```python
from build123d import *

# Parameters (mm, degrees)
CUT_EXTRUDE_2_DEPTH      = 0.5
PATTERN_CIRCULAR_1_COUNT = 2
PATTERN_CIRCULAR_1_ANGLE = 90
CUT_EXTRUDE_3_REACH      = 23.556
CUT_EXTRUDE_3_END_RADIUS = 6.5
SKETCH_4_R               = 0.85


with BuildPart() as part:
    # 草图1 → 旋转1 (revolve)
    with BuildSketch(Plane.XY, mode=Mode.PRIVATE) as revolve_1_sk:
        with BuildLine():
            Line((0, 0), (0, 2))
            Line((0, 2), (-20, 2))
            Line((-20, 2), (-20, 4))
            Line((-20, 4), (-21.524428901, 4))
            ThreePointArc((-21.524428901, 4), (-21.705500393, 3.956669476), (-21.847342271, 3.836065574))
            ThreePointArc((-21.847342271, 3.836065574), (-22.778904626, 2.017706029), (-23.1, 0))
            Line((-23.1, 0), (0, 0))
        make_face()
    revolve(revolve_1_sk.sketch.rotate(Axis((0, 0, 0), (-1, 0, 0)), 90), axis=Axis((0, 0, 0), (-1, 0, 0)))

    # 草图3 → 切除-拉伸2 (cut, symmetric)
    with BuildSketch(Plane.XY):
        Polygon((-20.8, -1), (-23.8, -2.495744824), (-23.8, 2.495744824), (-20.8, 1), align=None)
    cut_extrude_2 = extrude(amount=CUT_EXTRUDE_2_DEPTH, both=True, mode=Mode.SUBTRACT)

    # 阵列(圆周)1: 切除-拉伸2 ×2 about axis
    pattern_circular_1_axis = Axis((0, 0, 0), (1, 0, 0))
    for i in range(1, PATTERN_CIRCULAR_1_COUNT):
        add(cut_extrude_2.rotate(pattern_circular_1_axis, i * PATTERN_CIRCULAR_1_ANGLE / (PATTERN_CIRCULAR_1_COUNT - 1)), mode=Mode.SUBTRACT)

    # 切除-拉伸3: up to this sphere (the profile starts inside it)
    cut_extrude_3_end = Location((-16.6, 0, 0)) * Sphere(CUT_EXTRUDE_3_END_RADIUS, mode=Mode.PRIVATE)
    # 草图4 → 切除-拉伸3 (cut, up to the surface)
    with BuildSketch(Plane.ZY.offset(20.8), mode=Mode.PRIVATE) as cut_extrude_3_sk1:
        Circle(SKETCH_4_R)
    cut_extrude_3_tool1 = extrude(cut_extrude_3_sk1.sketch, amount=CUT_EXTRUDE_3_REACH, mode=Mode.PRIVATE) & cut_extrude_3_end
    add(cut_extrude_3_tool1.solids().sort_by_distance((-20.8, 0, 0))[0], mode=Mode.SUBTRACT)


solid = part.part
```
The model under review builds one solid part; all positions refer to its coordinate system, in mm. A direction names the side the tool comes from. Round coordinates to 2 decimals unless told otherwise and drop trailing zeros. Write each loop counter-clockwise with the first axis right and the second up, starting at its lowest first coordinate (ties: lowest second). Pieces come first, ordered by that corner, then holes. Notation, with made-up numbers: (38.5, -38.5) - (84.5, -38.5) arc R28 ccw to (84.5, -20.5) - close; hole circle Ø8 at (75.5, 67.25). An arc over 180 degrees is marked (long way). Answer as CSV lines item,"result". Start each with the question number.
(1) We need section A-A on z = 0. State the section outline as (x, y) points.
(2) We need section C-C on x = -9. State the section outline as (y, z) points, plus the area to 3 significant figures.
(3) For pin 1 Ø1 at (x, z) = (-21.5, 1) entering from +Y; pin 2 Ø1.5 at (x, y) = (-11, 1) entering from -Z; pin 3 Ø1.4 at (x, z) = (-21.5, -1.5) entering from -Y; pin 4 Ø1 at (x, y) = (-7, 3) entering from -Z (1 decimal), all flat-tipped, find the tip position at first contact; note any pin that passes through.
(4) To check wall thickness, follow line 1 (X direction, y = -0.75, z = -0.25); line 2 (X direction, y = -0.75, z = -3.25); line 3 (Y direction, x = -8.75, z = -0.5). State the ranges of each line that lie inside material, in increasing order.
(5) Draft analysis for pull direction Z (two halves, no side actions). For faces 1 (the flat face through (-22, -1, 0.5)), 2 (the flat face through (-21.8, 0, 1.5)), 3 (the flat face through (0, 0, 0)), 4 (the cylindrical face through (-20.773, 3.905, 0.867)), state which applies: pulls with the +Z half, pulls with the -Z half, needs draft (parallel to the pull), parting line crosses it, or undercut.
(6) For faces 5 (the cylindrical face through (-10, 2, 0)), 6 (the flat face through (-22, -0.5, 1)), list the 3-axis set-ups (+Z, -Z, +X, -X, +Y, -Y) from which the entire face can be reached by the end or side of a thin tool; tool diameter is ignored.
Worked answers:
1,outline,"(-22.79, -1.99) arc R6.5 ccw to (-21.85, -3.84) arc R0.4 ccw to (-21.52, -4) - (-20, -4) - (-20, -2) - (0, -2) - (0, 2) - (-20, 2) - (-20, 4) - (-21.52, 4) arc R0.4 ccw to (-21.85, 3.84) arc R6.5 ccw to (-22.79, 1.99) - (-20.8, 1) - (-20.8, -1) - close"
2,outline,"circle Ø4 at (0, 0)"
2,area,"12.6 mm²"
3,pin 1,"y = 3.97"
3,pin 2,"z = -1.98"
3,pin 3,"y = -3.92"
3,pin 4,"through"
4,line 1,"-20.8 to 0"
4,line 2,"-22.18 to -20"
4,line 3,"-1.94 to 1.94"
5,face 1,"undercut"
5,face 2,"undercut"
5,face 3,"needs draft"
5,face 4,"parting line crosses it"
6,face 5,"+X"
6,face 6,"-X"
